from build123d import *

# Parameters (mm, degrees)
BOSS_EXTRUDE1_DEPTH     = 2
SKETCH3_R               = 3
BOSS_EXTRUDE2_DEPTH     = 1
SKETCH4_R               = 3
BOSS_EXTRUDE3_DEPTH     = 1
SKETCH5_R               = 1
CUT_EXTRUDE5_DEPTH      = 1
CUT_EXTRUDE5_DEPTH_BACK = 3


with BuildPart() as part:
    # Sketch2 → Boss-Extrude1 (new body)
    with BuildSketch(Plane.XY):
        Polygon((-18, 0), (18, 0), (19.732050808, 1), (20.970146046, 1), (20.970146046, 2), (19.732050808, 2), (18, 1), (-18, 1), (-19.732050808, 2), (-20.970146046, 2), (-20.970146046, 1), (-19.732050808, 1), align=None)
    extrude(amount=BOSS_EXTRUDE1_DEPTH)

    # Sketch3 → Boss-Extrude2 (add)
    with BuildSketch(Plane(origin=(0, 2, 0), x_dir=(1, 0, 0), z_dir=(0, 1, 0))):
        with Locations((-22.732050808, -1)):
            Circle(SKETCH3_R)
    extrude(amount=-BOSS_EXTRUDE2_DEPTH)

    # Sketch4 → Boss-Extrude3 (add)
    with BuildSketch(Plane(origin=(0, 2, 0), x_dir=(1, 0, 0), z_dir=(0, 1, 0))):
        with Locations((22.732050808, -1)):
            Circle(SKETCH4_R)
    extrude(amount=-BOSS_EXTRUDE3_DEPTH)

    # Sketch5 → Cut-Extrude5 (cut, two sides)
    with BuildSketch(Plane(origin=(0, 2, 0), x_dir=(1, 0, 0), z_dir=(0, 1, 0))) as cut_extrude5_sk:
        with Locations((-22.732050808, -1)):
            Circle(SKETCH5_R)
        with Locations((22.732050808, -1)):
            Circle(SKETCH5_R)
    extrude(amount=CUT_EXTRUDE5_DEPTH, mode=Mode.SUBTRACT)
    extrude(cut_extrude5_sk.sketch, amount=-CUT_EXTRUDE5_DEPTH_BACK, mode=Mode.SUBTRACT)


solid = part.part
Check sheet for the modelled part. Datum: model origin and axes. Units: mm. A direction names the side the tool comes from. Round coordinates to 2 decimals unless told otherwise and drop trailing zeros. Loops run counter-clockwise (first coordinate to the right, second up) from the corner with the lowest first, then second, coordinate; pieces in that order, holes last.
1. Sectioned sample at A-A on y = 1.45. Record the boundary of the cut face in (x, z).
2. Sectioned sample at B-B on z = 1. Record the boundary of the cut face in (x, y).
3. Mould release check, pull along X, two halves, no side actions. Record for faces 1 (the flat face through (-22.8, 2, 2.3)), 2 (the flat face through (18.85, 0.49, 0.99)), 3 (the cylindrical face through (21.733, 1.507, 0.956)), 4 (the flat face through (18.88, 1.51, 0.99)): released by +X, released by -X, zero draft, split by the parting line, or undercut.
4. Gauge pin test, flat ends, axial feed: pin 1 Ø1.2 at (x, z) = (-22.73, 1) entering from -Y; pin 2 Ø2 at (x, z) = (4, -0.5) entering from +Y; pin 3 Ø3 at (x, z) = (-21.5, 1) entering from -Y; pin 4 Ø0.6 at (x, y) = (-2, 1) entering from -Z. Record the tip position at first contact, or that the pin passes through.
5. Sectioned sample at D-D on x = -17. Record the boundary of the cut face in (y, z), and give its area (3 significant figures).
6. Set-up check for faces 5 (the flat face through (22, 1, 0)), 6 (the flat face through (-22.8, 1, 2.3)), 7 (the cylindrical face through (-25.73, 1.51, 0.88)), 8 (the flat face through (0, 1, 1)): record each of +Z, -Z, +X, -X, +Y, -Y from which the full face is reachable in a straight line by a thin tool's end or side.
7. Scan lines: probe 1 along X at (y, z) = (1.45, 1); probe 2 along X at (y, z) = (1.35, 1); probe 3 along Z at (x, y) = (12.5, 0.25). Record each from-to range of solid material in increasing order.
8. Sectioned sample at C-C on z = -1.2. Record the boundary of the cut face in (x, y).
Recorded:
1. outline: (-19.9, 0) - (-18.78, 0) - (-18.78, 2) - (-19.9, 2) arc R3 ccw (long way) to start; (18.78, 0) - (19.9, 0) arc R3 ccw (long way) to (19.9, 2) - (18.78, 2) - close; hole circle Ø2 at (-22.73, 1); hole circle Ø2 at (22.73, 1)
2. outline: (-25.73, 1) - (-23.73, 1) - (-23.73, 2) - (-25.73, 2) - close; (-21.73, 1) - (-19.73, 1) - (-18, 0) - (18, 0) - (19.73, 1) - (21.73, 1) - (21.73, 2) - (19.73, 2) - (18, 1) - (-18, 1) - (-19.73, 2) - (-21.73, 2) - close; (23.73, 1) - (25.73, 1) - (25.73, 2) - (23.73, 2) - close
3. face 1: zero draft
3. face 2: released by +X
3. face 3: undercut
3. face 4: undercut
4. pin 1: passes through
4. pin 2: stops at y = 1
4. pin 3: stops at y = 1
4. pin 4: stops at z = 0
5. outline: (0, 0) - (1, 0) - (1, 2) - (0, 2) - close
5. area: 2.00 mm2
6. face 5: +Z, -Z, +X, -Y
6. face 6: +Z, -Z, -X, -Y
6. face 7: +Y, -Y
6. face 8: +Z, -Z, +Y
7. probe 1: x = -25.73 to -23.73, -21.73 to -18.78, 18.78 to 21.73, 23.73 to 25.73
7. probe 2: x = -25.73 to -23.73, -21.73 to -18.61, 18.61 to 21.73, 23.73 to 25.73
7. probe 3: z = 0 to 2
8. outline: (-24.77, 1) - (-20.69, 1) - (-20.69, 2) - (-24.77, 2) - close; (20.69, 1) - (24.77, 1) - (24.77, 2) - (20.69, 2) - close
